Geometry check sheet. Reference: the model listing, model coordinates, mm. Face numbers are marked on the shaded views. Give positions to 0.01 mm unless a question says otherwise; leave off trailing zeros. Order: outer loops, then holes, each group sorted by start corner. A loop starts at its lowest first (then second) coordinate and runs counter-clockwise, first axis right, second up.
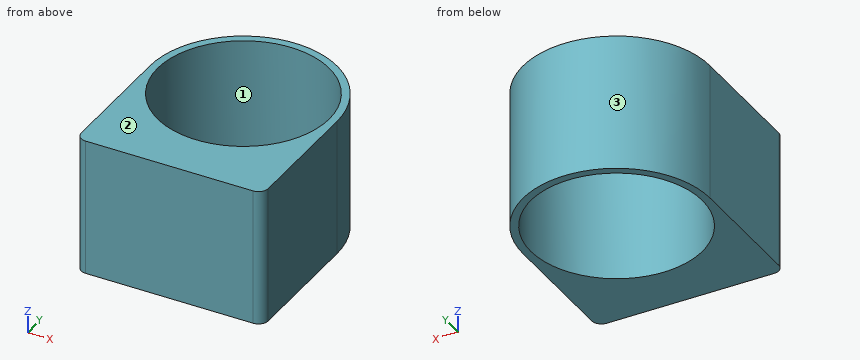
Autodesk Fusion 360 part; units mm, degrees
sketch "Sketch1" plane through (0, 0, 0) normal (0, 0, 1) x (1, 0, 0)
  line L0 (6.5, -1.7) -> (-6.5, -1.7)
  line L1 (-6.5, -1.7) -> (-6.5, 1.7)
  line L2 (-6.5, 1.7) -> (6.5, 1.7)
  line L3 (6.5, 1.7) -> (6.5, -1.7)
  line L4 (6.5, -1.7) -> (-6.5, 1.7) construction
  line L5 (-6.5, -1.7) -> (6.5, 1.7) construction
  line L6 (6.5, -2.3) -> (-6.5, -2.3)
  line L7 (6.5, -2.3) -> (9.65, -2.3)
  circle A0 centre (0, 11.55) radius 8.85
  line L8 (9.65, -2.3) -> (9.65, 11.55)
  line L9 (0, 2.5) -> (0, 20)
  line L10 (-6.5, -2.3) -> (-9.65, -2.3)
  line L11 (-9.65, -2.3) -> (-9.65, 11.55)
  arc A1 (9.65, 11.55) -> (-9.65, 11.55) centre (0, 11.55) ccw
  dimension "d1" = 13
  dimension "d2" = 3.4
  dimension "d3" = -0.6
  dimension "d4" = 17.7
  dimension "d5" = 1
  dimension "d6" = 0.8
extrude "Extrude1" add sketch "Sketch1" along normal blind 0.4 contours L0 L1 L2 L3 | L6 L7 L8 L10 L11 A1
extrude "Extrude2" add sketch "Sketch1" along normal blind 13 from surface at 0.4
extrude "Extrude3" add sketch "Sketch1" along normal blind 0.8 from surface at 13.4 contours L0 L1 L2 L3 | L6 L7 L8 L10 L11 A1
fillet "Fillet1" radius 1 2 edges at (9.65, -2.3, 7.1) (-9.65, -2.3, 7.1)
Q1. Thickness scan on L1, parallel to Y at x = 0, z = 11; L2, parallel to Z at x = 2.25, y = 1; L3, parallel to Y at x = 5.75, z = 8.25. Record the ranges inside material, lowest first.
Q2. Cross-section at A-A, the plane x = 0. Record the boundary of the cut face in (y, z).
Q3. Cross-section at C-C, the plane y = 3.5. Record the boundary of the cut face in (x, z).
Q4. Release check for a two-part mould opening along X. For the marked faces 1, 2 and 3 record: pulls with the +X half, pulls with the -X half, needs draft (parallel to the pull), parting line crosses it, or undercut.
Q5. Cross-section at D-D, the plane x = -8.25. Record the boundary of the cut face in (y, z), and give its area (3 significant figures).
Q6. Cross-section at B-B, the plane z = 7.5. Record the boundary of the cut face in (x, y).
Q7. Gauge pin test, flat ends, axial feed: P1, Ø3.5, axis at x = 0, y = 0, coming from the -Z side; P2, Ø6, axis at y = 17, z = 10, coming from the -X side. Record the tip position at first contact, or that the pin passes through.
Answers follow:
1. L1: y = -2.3 to -1.7, 1.7 to 2.7, 20.4 to 21.2
1. L2: z = 0 to 0.4, 13.4 to 14.2
1. L3: y = -2.3 to -1.7, 1.7 to 4.82, 18.28 to 19.3
2. outline: (-2.3, 0) - (2.7, 0) - (2.7, 14.2) - (-2.3, 14.2) - close; (20.4, 0) - (21.2, 0) - (21.2, 14.2) - (20.4, 14.2) - close; hole (-1.7, 0.4) - (1.7, 0.4) - (1.7, 13.4) - (-1.7, 13.4) - close
3. outline: (-9.65, 0) - (-3.68, 0) - (-3.68, 14.2) - (-9.65, 14.2) - close; (3.68, 0) - (9.65, 0) - (9.65, 14.2) - (3.68, 14.2) - close
4. face 1: undercut
4. face 2: needs draft
4. face 3: parting line crosses it
5. outline: (-2.3, 0) - (8.35, 0) - (8.35, 14.2) - (-2.3, 14.2) - close; (14.75, 0) - (16.56, 0) - (16.56, 14.2) - (14.75, 14.2) - close
5. area: 177 mm2
6. outline: (-9.65, -1.3) arc R1 ccw to (-8.65, -2.3) - (8.65, -2.3) arc R1 ccw to (9.65, -1.3) - (9.65, 11.55) arc R9.65 ccw to (-9.65, 11.55) - close; hole circle Ø17.7 at (0, 11.55); hole (-6.5, -1.7) - (6.5, -1.7) - (6.5, 1.7) - (-6.5, 1.7) - close
7. P1: stops at z = 0
7. P2: stops at x = -9.33
